from build123d import *

# Parameters (mm, degrees)
SKETCH1_R                = 79.375
SKETCH1_R_2              = 39.624
BOSS_EXTRUDE1_DEPTH      = 1.5875
SKETCH2_R                = 79.375
SKETCH2_R_2              = 45.974
CUT_EXTRUDE1_DEPTH       = 2.5875
BOSS_EXTRUDE2_DEPTH      = 1.5875
FILLET1_R                = 6.35
CIRPATTERN1_COUNT        = 4
FILLET1_OF_CIRPATTERN1_R = 6.35


with BuildPart() as part:
    # Sketch1 → Boss-Extrude1 (new body)
    with BuildSketch(Plane.XY):
        Circle(SKETCH1_R)
        Circle(SKETCH1_R_2, mode=Mode.SUBTRACT)
    extrude(amount=BOSS_EXTRUDE1_DEPTH)

    # Sketch2 → Cut-Extrude1 (cut, through all)
    with BuildSketch(Plane.XY.offset(1.5875)):
        Circle(SKETCH2_R)
        Circle(SKETCH2_R_2, mode=Mode.SUBTRACT)
    extrude(amount=-CUT_EXTRUDE1_DEPTH, mode=Mode.SUBTRACT)

    # Sketch3 → Boss-Extrude2 (add)
    with BuildSketch(Plane.XY.offset(1.5875)):
        with BuildLine():
            ThreePointArc((30.375497444, 73.332937893), (0, 79.375), (-30.375497444, 73.332937893))
            Line((-30.375497444, 73.332937893), (-17.59348812, 42.474437628))
            ThreePointArc((-17.59348812, 42.474437628), (0, 45.974), (17.59348812, 42.474437628))
            Line((17.59348812, 42.474437628), (30.375497444, 73.332937893))
        make_face()
    boss_extrude2 = extrude(amount=-BOSS_EXTRUDE2_DEPTH)

    # Fillet1
    fillet1_edges = [part.edges().sort_by_distance(p)[0] for p in [
        (17.59348812, 42.474437628, 0.79375),
        (-17.59348812, 42.474437628, 0.79375),
    ]]
    fillet(fillet1_edges, radius=FILLET1_R)

    # CirPattern1: Boss-Extrude2 ×4 about axis
    cirpattern1_axis = Axis((0, 0, 0), (0, 0, 1))
    for i in range(1, CIRPATTERN1_COUNT):
        add(boss_extrude2.rotate(cirpattern1_axis, i * 360 / CIRPATTERN1_COUNT))

    # Fillet1 of CirPattern1
    fillet1_of_cirpattern1_edges = [part.edges().sort_by_distance(p)[0] for p in [
        (-42.474437628, 17.59348812, 0.79375),
        (-42.474437628, -17.59348812, 0.79375),
        (-17.59348812, -42.474437628, 0.79375),
        (17.59348812, -42.474437628, 0.79375),
        (42.474437628, -17.59348812, 0.79375),
        (42.474437628, 17.59348812, 0.79375),
    ]]
    fillet(fillet1_of_cirpattern1_edges, radius=FILLET1_OF_CIRPATTERN1_R)


solid = part.part
Can you work these out from the model? Positions are in its coordinate system, mm. A direction names the side the tool comes from. Coordinates: 2 decimals unless noted, no trailing zeros. Write each loop counter-clockwise with the first axis right and the second up, starting at its lowest first coordinate (ties: lowest second). Pieces come first, ordered by that corner, then holes. Notation, with made-up numbers: (-13.75, 77) - (19.25, 77) arc R15 cw to (19.25, 106) - close; hole circle Ø2 at (89.25, 48.5). An arc over 180 degrees is marked (long way). Return JSON: item names as keys, results as strings. Group by question number.
Item 1: Please list where these lines run through material, in increasing order: probe 1 along Y at (x, z) = (0, 0.85) (3 decimals); probe 2 along X at (y, z) = (-25.5, 0.95); probe 3 along X at (y, z) = (24, 1.1).
Item 2: If we section it at A-A (x = 0): Write out the boundary of the cut face in (y, z) (1 decimal), then the cut area to 3 significant figures.
Item 3: If we section it at D-D (x = 45.5): Write out the boundary of the cut face in (y, z).
Item 4: Which directions (+Z, -Z, +X, -X, +Y, -Y) give clear straight access to the entire face, cutting with the end or side of a thin tool? Please do faces 1 (the face through (-60.84, -25.2, 0.8)), 2 (the face through (-25.2, 60.84, 0.8)), 3 (the face through (25.05, 60.48, 0.8)).
Item 5: We'd pull the mould along X, two halves only. Please class faces 4 (the face through (-60.48, 25.05, 0.8)), 5 (the face through (60.84, 25.2, 0.8)), 6 (the face through (-25.05, -60.48, 0.8)), 7 (the face through (0.436, 79.374, 0.805)): pulls with the +X half, pulls with the -X half, needs draft (parallel to the pull), parting line crosses it, or undercut.
Return value:
{
 "1": {"probe 1": "y = -79.375 to -39.624, 39.624 to 79.375", "probe 2": "x = -75.17 to -61.56, -38.25 to -30.33, 30.33 to 38.25, 61.56 to 75.17", "probe 3": "x = -75.66 to -57.94, -39.21 to -31.53, 31.53 to 39.21, 57.94 to 75.66"},
 "2": {"outline": "(-79.4, 0) - (-39.6, 0) - (-39.6, 1.6) - (-79.4, 1.6) - close; (39.6, 0) - (79.4, 0) - (79.4, 1.6) - (39.6, 1.6) - close", "area": "126 mm^2"},
 "3": {"outline": "(-19.39, 0) - (19.39, 0) - (19.39, 1.59) - (-19.39, 1.59) - close"},
 "4": {"face 1": "+Z, -Z, -Y", "face 2": "+Z, -Z, -X", "face 3": "+Z, -Z, +X"},
 "5": {"face 4": "undercut", "face 5": "undercut", "face 6": "pulls with the -X half", "face 7": "parting line crosses it"}
}
